Geometry check sheet. Reference: the model listing, model coordinates, mm. A direction names the side the tool comes from. Give positions to 0.01 mm unless a question says otherwise; leave off trailing zeros. Write each loop counter-clockwise with the first axis right and the second up, starting at its lowest first coordinate (ties: lowest second). Pieces come first, ordered by that corner, then holes. Notation, with made-up numbers: (-1, -21) -> (52, -21) arc R28 ccw to (52, 9) -> close; hole circle Ø2 at (-39, 18). An arc over 180 degrees is marked (long way). Write item = value, one per line. Start each with the question number.
1. Set-up check for faces 1 (the flat face through (1, 0, -1)), 2 (the flat face through (-40, 50, -14)): record each of +Z, -Z, +X, -X, +Y, -Y from which the full face is reachable in a straight line by a thin tool's end or side.
2. Thickness scan on line 1 along Y through (x, z) = (40.5, -8.5); line 2 along X through (y, z) = (18, 0); line 3 along Y through (x, z) = (-2, 20.5). Record the ranges inside material, lowest first.
3. Cross-section at A-A, the plane y = 22. Record the cut outline in (x, z).
4. Mould release check, pull along Z, two halves, no side actions. Record for faces 3 (the cylindrical face through (-17.235, 24.65, 41.569)), 4 (the flat face through (28, 60, -28)), 5 (the flat face through (1, 6, -1)): pulls with the +Z half, pulls with the -Z half, needs draft (parallel to the pull), parting line crosses it, or undercut.
5. Depth check by flat-ended pin: P1, Ø10, axis at x = -23.5, z = 0, coming from the +Y side; P2, Ø5, axis at y = 11, z = 31.5, coming from the +X side; P3, Ø12, axis at x = -3, y = 50.5, coming from the -Z side; P4, Ø4, axis at y = 12.5, z = -26, coming from the +X side. Enter the tip coordinate at first touch or a pass-through.
```python
from build123d import *
from build123d.topology import SkipClean

# Parameters (mm, degrees)
SKETCH1_R           = 45
BOSS_EXTRUDE1_DEPTH = 50
SHELL1_T            = -6
SKETCH3_W           = 3
SKETCH3_H           = 10
THREAD1_PITCH       = 3


with BuildPart() as part:
    # Sketch1 → Boss-Extrude1 (new body)
    with BuildSketch(Plane(origin=(0, 0, 0), x_dir=(1, 0, 0), z_dir=(0, 1, 0))):
        with Locations(Location((0, 0, 0), (0, 0, 270))):
            Circle(SKETCH1_R)
    extrude(amount=BOSS_EXTRUDE1_DEPTH)

    # Shell1
    shell1_openings = [part.faces().sort_by_distance(p)[0] for p in [
        (0, 50, 0),
    ]]
    offset(amount=SHELL1_T, openings=shell1_openings, kind=Kind.INTERSECTION)

    # Sketch3 → Revolve1 (revolve)
    with SkipClean():  # the faces are left unmerged after this step: merging them gives an invalid solid
        with BuildSketch(Plane.XY, mode=Mode.PRIVATE) as revolve1_sk:
            with Locations((-40.5, 55)):
                Rectangle(SKETCH3_W, SKETCH3_H)
        revolve(revolve1_sk.sketch.rotate(Axis((0, 0, 0), (0, 1, 0)), 270), axis=Axis((0, 0, 0), (0, 1, 0)))
    add(part.part.scale(1), mode=Mode.REPLACE)  # the faces are merged on a copy

    # Thread1: the profile of Thread Profile1 profile screwed along a right-hand helix of 2.666667 turns, 10 arcs to a turn; built about Z, then put on its axis
    thread1_z = Axis((0, 0, 0), (0, 0, 1))
    thread1_corners = [(42.0003, 0, -0.000173205), (42.0003, 0, 2.625173197), (40.376202375, 0, 1.687499996), (40.376202375, 0, 0.937499996)]
    with BuildLine(mode=Mode.PRIVATE) as thread1_profile:
        Line(thread1_corners[0], thread1_corners[1])
        Line(thread1_corners[1], thread1_corners[2])
        Line(thread1_corners[2], thread1_corners[3])
        Line(thread1_corners[3], thread1_corners[0])
    thread1_cap = Face(thread1_profile.wire())
    thread1_turn_angles = [0, 18, 36, 54, 72, 90, 108, 126, 144, 162, 180, 198, 216, 234, 252, 270, 288, 306, 324, 342, 360]
    thread1_turn_weights = [1, 0.9510565162951535, 1, 0.9510565162951535, 1, 0.9510565162951535, 1, 0.9510565162951535, 1, 0.9510565162951535, 1, 0.9510565162951535, 1, 0.9510565162951535, 1, 0.9510565162951535, 1, 0.9510565162951535, 1, 0.9510565162951535, 1]
    thread1_turn_rails = [Edge.make_bspline([Vector(p[0], p[1], 0).rotate(thread1_z, thread1_turn_angles[k]) / thread1_turn_weights[k] + Vector(0, 0, p[2] + THREAD1_PITCH * thread1_turn_angles[k] / 360) for k in range(21)], [0, 0, 0, 1, 1, 2, 2, 3, 3, 4, 4, 5, 5, 6, 6, 7, 7, 8, 8, 9, 9, 10, 10, 10], 2, thread1_turn_weights) for p in thread1_corners]
    thread1_turn_sides = [Face.make_surface_from_curves(thread1_turn_rails[p[0]], thread1_turn_rails[p[1]]) for p in [(0, 1), (1, 2), (2, 3), (3, 0)]]
    thread1_last_angles = [720, 738, 756, 774, 792, 810, 828, 846, 864, 882, 900, 918, 936, 948, 960]
    thread1_last_weights = [1, 0.9510565162951535, 1, 0.9510565162951535, 1, 0.9510565162951535, 1, 0.9510565162951535, 1, 0.9510565162951535, 1, 0.9510565162951535, 1, 0.978147600733806, 1]
    thread1_last_rails = [Edge.make_bspline([Vector(p[0], p[1], 0).rotate(thread1_z, thread1_last_angles[k]) / thread1_last_weights[k] + Vector(0, 0, p[2] + THREAD1_PITCH * thread1_last_angles[k] / 360) for k in range(15)], [0, 0, 0, 1, 1, 2, 2, 3, 3, 4, 4, 5, 5, 6, 6, 7, 7, 7], 2, thread1_last_weights) for p in thread1_corners]
    thread1_last_sides = [Face.make_surface_from_curves(thread1_last_rails[p[0]], thread1_last_rails[p[1]]) for p in [(0, 1), (1, 2), (2, 3), (3, 0)]]
    thread1 = Plane(origin=(0, 60, 0), x_dir=(-1, 0, 0), z_dir=(0, -1, 0)) * Solid(Shell([*[p.moved(Location((0, 0, THREAD1_PITCH * i))) for i in range(2) for p in thread1_turn_sides], *thread1_last_sides, thread1_cap, thread1_cap.rotate(thread1_z, 960).moved(Location((0, 0, THREAD1_PITCH * 960 / 360)))]))
    add(thread1, mode=Mode.SUBTRACT)


solid = part.part
```
Answers:
q1.face_1 = +Z, -Z, +X, -X, -Y
q1.face_2 = +Y
q2.line_1 = 0 to 50.33, 52.24 to 53.33, 55.24 to 56.33, 58.24 to 60
q2.line_2 = -45 to -39, 39 to 45
q2.line_3 = 0 to 6
q3.outline = circle Ø90 at (0, 0); hole circle Ø78 at (0, 0)
q4.face_3 = parting line crosses it
q4.face_4 = needs draft
q4.face_5 = undercut
q5.P1 = 6
q5.P2 = 34.41
q5.P3 = -45
q5.P4 = 38.07
